Design review of the part built by this model. Coordinates are the model's own, in mm. A direction names the side the tool comes from. Give positions to 0.01 mm unless a question says otherwise; leave off trailing zeros. Loops run counter-clockwise (first coordinate to the right, second up) from the corner with the lowest first, then second, coordinate; pieces in that order, holes last. Notation, with made-up numbers: (49.25, 23) - (86.25, 23) arc R27 ccw to (86.25, 44) - close; hole circle Ø6 at (36, -26.5). An arc over 180 degrees is marked (long way). One line per item, written item: value. Start each with the question number.
Autodesk Inventor part; units mm, degrees
ref_plane "YZ Plane" through (0, 0, 0) normal (1, 0, 0) x (0, 1, 0)
ref_plane "XZ Plane" through (0, 0, 0) normal (0, 1, 0) x (-1, 0, 0)
ref_plane "XY Plane" through (0, 0, 0) normal (0, 0, 1) x (1, 0, 0)
sketch "Schizzo1" plane through (0, 0, 0) normal (0, 0, 1) x (1, 0, 0)
  line L0 (0, 0) -> (0, 24.2842) construction
  line L1 (-25, 0) -> (-25, 10)
  line L2 (-25, 10) -> (-21.85, 10)
  line L3 (-21.85, 10) -> (-21.85, 14.5)
  line L4 (-21.85, 14.5) -> (-25, 14.5)
  line L5 (-25, 14.5) -> (-25, 24)
  line L6 (-25, 24) -> (-37.5, 24)
  line L7 (-37.5, 24) -> (-37.5, 34)
  line L8 (-37.5, 34) -> (-22.5, 34)
  line L9 (-22.5, 34) -> (-22.5, 40)
  line L10 (-22.5, 40) -> (-4, 40)
  line L11 (-4, 40) -> (-4, 32)
  line L12 (-4, 32) -> (-15, 32)
  line L13 (-15, 32) -> (-15, 0)
  line L14 (-25, 0) -> (-15, 0)
  dimension "d0" = 30
  dimension "d1" = 8
  dimension "d2" = 43.7
  dimension "d3" = 50
  dimension "d4" = 45
  dimension "d5" = 75
  dimension "d9" = 24
  dimension "d10" = 34
  dimension "d11" = 32
  dimension "d13" = 4.5
  dimension "d14" = 10
  dimension "d15" = 40
revolve "Rivoluzione1" add sketch "Schizzo1" angle 360 about axis through (0, 0, 0) along (0, 1, 0)
sketch "Schizzo2" plane through (0, 34, 0) normal (0, 1, 0) x (1, 0, 0)
  circle A0 centre (0, 0) radius 25
  circle A1 centre (0, 0) radius 30 construction
  circle A2 centre (30, 0) radius 3.496
  circle A3 centre (0, 30) radius 2.9704
  circle A4 centre (-30, 0) radius 3.7285
  circle A5 centre (0, -30) radius 3.043
  circle A6 centre (-21.2132, -21.2132) radius 2.9112
  circle A7 centre (21.2132, 21.2132) radius 2.3494
  dimension "d17" = 60
  dimension "d18" = 45
  dimension "d19" = 45
hole "Foro1" at (-30, 34, 0) at (0, 34, -30) at (30, 34, 0) at (0, 34, 30) direction (0, -1, 0) diameter 5.5 end through all counterbore diameter 10 counterbore depth 5
hole "Foro2" at (21.2132, 34, -21.2132) at (-21.2132, 34, 21.2132) direction (0, -1, 0) diameter 5 end through all
properties part number "05-16-2023 Pompa Manuale OLIO"
(1) Take a section at C-C on y = 5.5. State the section outline as (x, z) points, and give its area (3 significant figures).
(2) Take a section at D-D on y = 25. State the section outline as (x, z) points.
(3) For pin 1 Ø3 at (x, z) = (-21.21, 21.21) entering from +Y; pin 2 Ø3 at (y, z) = (14, -5) entering from -X; pin 3 Ø2 at (x, y) = (-26.5, 32.5) entering from +Z; pin 4 Ø4 at (y, z) = (25, 29) entering from +X, all flat-tipped, find the tip position at first contact; note any pin that passes through.
(4) Draft analysis for pull direction X (two halves, no side actions). For faces 1 (the cylindrical face through (-23.846, 19.316, 7.509)), 2 (the cylindrical face through (22.171, 28.93, -18.904)), 3 (the flat face through (0.1, 14.5, -22.1)), state which applies: pulls with the +X half, pulls with the -X half, needs draft (parallel to the pull), parting line crosses it, or undercut.
(5) To check wall thickness, follow L1, parallel to Z at x = 0, y = 25.25; L2, parallel to X at y = 30.9, z = 30; L3, parallel to X at y = 28.5, z = 2. State the ranges of each line that lie inside material, in increasing order. Write a range as from..to.
(6) Take a section at B-B on z = -29. State the section outline as (x, y) points, and give its area (3 significant figures).
(7) Take a section at A-A on x = -30. State the section outline as (y, z) points, and give its area (4 significant figures).
(8) Machinability: for faces 4 (the flat face through (-24, 24, -8)), 5 (the cylindrical face through (27.273, 26.465, -0.358)), 6 (the flat face through (32.2, 29, 2.2)), which of the approach directions +Z, -Z, +X, -X, +Y, -Y give a long, thin tool a straight path to every point of the face, cutting with its end or side? Answer none if there is none.
Here are the results:
1. outline: circle Ø50 at (0, 0); hole circle Ø30 at (0, 0)
1. area: 1,260 mm²
2. outline: circle Ø75 at (0, 0); hole circle Ø5.5 at (-30, 0); hole circle Ø5 at (-21.21, 21.21); hole circle Ø30 at (0, 0); hole circle Ø5.5 at (0, -30); hole circle Ø5.5 at (0, 30); hole circle Ø5 at (21.21, -21.21); hole circle Ø5.5 at (30, 0)
3. pin 1: through
3. pin 2: x = -24.74
3. pin 3: z = 27.5
3. pin 4: x = 26.02
4. face 1: parting line crosses it
4. face 2: undercut
4. face 3: needs draft
5. L1: -37.5..-32.75, -27.25..-15, 15..27.25, 32.75..37.5
5. L2: -22.5..-5, 5..22.5
5. L3: -37.45..-31.89, -28.11..-14.87, 14.87..28.11, 31.89..37.45
6. outline: (-23.77, 24) - (-2.56, 24) - (-2.56, 29) - (-4.9, 29) - (-4.9, 34) - (-23.77, 34) - close; (2.56, 24) - (23.77, 24) - (23.77, 34) - (4.9, 34) - (4.9, 29) - (2.56, 29) - close
6. area: 401 mm²
7. outline: (24, -22.5) - (34, -22.5) - (34, -5) - (29, -5) - (29, -2.75) - (24, -2.75) - close; (24, 2.75) - (29, 2.75) - (29, 5) - (34, 5) - (34, 22.5) - (24, 22.5) - close
7. area: 372.5 mm²
8. face 4: -Y
8. face 5: +Y, -Y
8. face 6: +Y
